Geometry: final body of the model. Coordinates: model frame, mm. Give positions to 0.01 mm unless a question says otherwise; leave off trailing zeros. Loops run counter-clockwise (first coordinate to the right, second up) from the corner with the lowest first, then second, coordinate; pieces in that order, holes last. Notation, with made-up numbers: (-26.75, 34.25) - (11.25, 34.25) arc R23 cw to (11.25, 49.25) - close; hole circle Ø5 at (65, 67). An arc over 180 degrees is marked (long way). Use one line per item in the form item = value.
Autodesk Inventor part; units mm, degrees
ref_plane "YZ Plane" through (0, 0, 0) normal (1, 0, 0) x (0, 1, 0)
ref_plane "XZ Plane" through (0, 0, 0) normal (0, 1, 0) x (-1, 0, 0)
ref_plane "XY Plane" through (0, 0, 0) normal (0, 0, 1) x (1, 0, 0)
sketch "Skizze1" plane through (0, 0, 0) normal (0, 0, 1) x (1, 0, 0)
  line L0 (0, 0) -> (90.4, 0)
  line L1 (90.4, 0) -> (90.4, 80)
  line L2 (90.4, 80) -> (0, 80)
  line L3 (0, 80) -> (0, 0)
  line L4 (2.6, 69.1) -> (87.8, 69.1) construction
  line L5 (87.8, 69.1) -> (87.8, 10.9) construction
  line L6 (87.8, 10.9) -> (2.6, 10.9) construction
  line L7 (2.6, 10.9) -> (2.6, 69.1) construction
  circle A0 centre (2.6, 69.1) radius 1.6
  circle A1 centre (2.6, 10.9) radius 1.6
  circle A2 centre (87.8, 69.1) radius 1.6
  circle A3 centre (87.8, 10.9) radius 1.6
  line L8 (25.2, 40) -> (65.2, 40) construction
  line L9 (65.2, 69.1) -> (65.2, 10.9) construction
  line L10 (65.2, 10.9) -> (47.65, 10.9) construction
  line L11 (65.2, 69.1) -> (82.75, 69.1) construction
  line L12 (25.2, 69.1) -> (25.2, 10.9) construction
  line L13 (25.2, 69.1) -> (42.75, 69.1) construction
  line L14 (25.2, 10.9) -> (7.65, 10.9) construction
  circle A4 centre (7.65, 10.9) radius 1.225
  circle A5 centre (42.75, 69.1) radius 1.225
  circle A6 centre (82.75, 69.1) radius 1.225
  circle A7 centre (47.65, 10.9) radius 1.225
  circle A8 centre (47.65, 77.32) radius 1.195
  circle A9 centre (42.75, 2.68) radius 1.195
  circle A10 centre (65.2, 10.9) radius 1.6
  circle A11 centre (65.2, 69.1) radius 1.6
  circle A12 centre (25.2, 69.1) radius 1.6
  circle A13 centre (25.2, 10.9) radius 1.6
  line L15 (1.9, 19.45) -> (3.9, 19.45) construction
  line L16 (3.9, 19.45) -> (3.9, 17.45) construction
  line L17 (3.9, 17.45) -> (1.9, 17.45) construction
  line L18 (1.9, 17.45) -> (1.9, 19.45) construction
  line L19 (1.9, 25.15) -> (3.9, 25.15) construction
  line L20 (3.9, 25.15) -> (3.9, 23.15) construction
  line L21 (3.9, 23.15) -> (1.9, 23.15) construction
  line L22 (1.9, 23.15) -> (1.9, 25.15) construction
  line L23 (1.8, 30.1) -> (4.2, 30.1) construction
  line L24 (4.2, 30.1) -> (4.2, 27.9) construction
  line L25 (4.2, 27.9) -> (1.8, 27.9) construction
  line L26 (1.8, 27.9) -> (1.8, 30.1) construction
  line L27 (2.9, 19.45) -> (2.9, 23.15) construction
  circle A14 centre (1.9, 23.15) radius 0.5588
  circle A15 centre (3.9, 23.15) radius 0.5588
  circle A16 centre (3.9, 25.15) radius 0.5588
  circle A17 centre (1.9, 25.15) radius 0.5588
  circle A18 centre (1.9, 19.45) radius 0.5588
  circle A19 centre (3.9, 19.45) radius 0.5588
  circle A20 centre (3.9, 17.45) radius 0.5588
  circle A21 centre (1.9, 17.45) radius 0.5588
  line L28 (1.8, 27.9) -> (4.2, 30.1) construction
  circle A22 centre (4.2, 27.9) radius 0.4064
  circle A23 centre (1.8, 27.9) radius 0.4064
  circle A24 centre (4.2, 30.1) radius 0.4064
  circle A25 centre (1.8, 30.1) radius 0.4064
  line L29 (86.3, 19.45) -> (88.3, 19.45) construction
  line L30 (88.3, 19.45) -> (88.3, 17.45) construction
  line L31 (88.3, 17.45) -> (86.3, 17.45) construction
  line L32 (86.3, 17.45) -> (86.3, 19.45) construction
  line L33 (86.3, 25.15) -> (88.3, 25.15) construction
  line L34 (88.3, 25.15) -> (88.3, 23.15) construction
  line L35 (88.3, 23.15) -> (86.3, 23.15) construction
  line L36 (86.3, 23.15) -> (86.3, 25.15) construction
  line L37 (87.3, 19.45) -> (87.3, 23.15) construction
  circle A26 centre (86.3, 23.15) radius 0.5588
  circle A27 centre (88.3, 23.15) radius 0.5588
  circle A28 centre (88.3, 25.15) radius 0.5588
  circle A29 centre (86.3, 25.15) radius 0.5588
  circle A30 centre (86.3, 19.45) radius 0.5588
  circle A31 centre (88.3, 19.45) radius 0.5588
  circle A32 centre (88.3, 17.45) radius 0.5588
  circle A33 centre (86.3, 17.45) radius 0.5588
  line L38 (55.65, 77.61) -> (74.75, 77.61) construction
  line L39 (74.75, 77.61) -> (74.75, 2.39) construction
  line L40 (74.75, 2.39) -> (55.65, 2.39) construction
  line L41 (55.65, 2.39) -> (55.65, 77.61) construction
  circle A34 centre (55.65, 2.39) radius 0.66
  circle A35 centre (74.75, 2.39) radius 0.66
  circle A36 centre (74.75, 77.61) radius 0.66
  circle A37 centre (55.65, 77.61) radius 0.66
  line L42 (15.65, 77.61) -> (34.75, 77.61) construction
  line L43 (34.75, 77.61) -> (34.75, 2.39) construction
  line L44 (34.75, 2.39) -> (15.65, 2.39) construction
  line L45 (15.65, 2.39) -> (15.65, 77.61) construction
  circle A38 centre (15.65, 2.39) radius 0.66
  circle A39 centre (34.75, 2.39) radius 0.66
  circle A40 centre (34.75, 77.61) radius 0.66
  circle A41 centre (15.65, 77.61) radius 0.66
  line L46 (55.65, 2.39) -> (74.75, 77.61) construction
  line L47 (15.65, 2.39) -> (34.75, 77.61) construction
  line L48 (23.2, 29.27) -> (23.2, 26.73) construction
  circle A42 centre (23.2, 26.73) radius 0.45
  circle A43 centre (23.2, 29.27) radius 0.45
  line L49 (27.2, 29.27) -> (27.2, 26.73) construction
  circle A44 centre (27.2, 26.73) radius 0.45
  circle A45 centre (27.2, 29.27) radius 0.45
  line L50 (23.2, 28) -> (27.2, 28) construction
  line L51 (63.2, 29.27) -> (63.2, 26.73) construction
  circle A46 centre (63.2, 26.73) radius 0.45
  circle A47 centre (63.2, 29.27) radius 0.45
  circle A48 centre (67.2, 29.27) radius 0.45
  line L52 (67.2, 29.27) -> (67.2, 26.73) construction
  circle A49 centre (67.2, 26.73) radius 0.45
  line L53 (63.2, 28) -> (67.2, 28) construction
  point P0 (2.9, 21.3)
  point P1 (3, 29)
  point P2 (87.3, 21.3)
  dimension "d0" = 90.4
  dimension "d1" = 80
  dimension "d2" = 2.6
  dimension "d3" = 10.9
  dimension "d4" = 69.1
  dimension "d5" = 87.8
  dimension "d6" = 3.2
  dimension "d7" = 40
  dimension "d8" = 25.2
  dimension "d9" = 65.2
  dimension "d10" = 2.45
  dimension "d11" = 2.39
  dimension "d12" = 17.55
  dimension "d13" = 17.55
  dimension "d14" = 37.32
  dimension "d15" = 37.32
  dimension "d16" = 3.2
  dimension "d17" = 29.1
  dimension "d18" = 17.55
  dimension "d21" = 1.85
  dimension "d22" = 2
  dimension "d23" = 1.1176
  dimension "d24" = 2.4
  dimension "d25" = 2.2
  dimension "d26" = 0.8128
  dimension "d27" = 1.85
  dimension "d28" = 2
  dimension "d29" = 1.1176
  dimension "d30" = 2.9
  dimension "d31" = 3
  dimension "d32" = 21.3
  dimension "d33" = 29
  dimension "d34" = 87.3
  dimension "d35" = 21.3
  dimension "d36" = 1.32
  dimension "d37" = 19.1
  dimension "d38" = 75.22
  dimension "d39" = 1.32
  dimension "d40" = 19.1
  dimension "d41" = 75.22
  dimension "d42" = 0.9
  dimension "d43" = 2.54
  dimension "d44" = 0.9
  dimension "d45" = 2.54
  dimension "d46" = 4
  dimension "d47" = 0.9
  dimension "d48" = 2.54
  dimension "d49" = 0.9
  dimension "d50" = 2.54
  dimension "d51" = 4
  dimension "d52" = 28
  dimension "d53" = 23.2
  dimension "d54" = 63.2
extrude "Extrusion1" add sketch "Skizze1" along normal mid plane 1.6
sketch "Skizze2" plane through (0, 0, 0.8) normal (0, 0, 1) x (1, 0, 0)
  line L0 (0, 79.9165) -> (90.4, 79.9165) construction
  line L1 (90.4, 79.9165) -> (90.4, 0.0835) construction
  line L2 (90.4, 0.0835) -> (0, 0.0835) construction
  line L3 (0, 0.0835) -> (0, 79.9165) construction
  point P0 (90.4, 40)
  point P1 (0, 40)
decal "Aufkleber1"
equation "\"d13\" = d12"
equation "\"d15\" = d14"
properties part number "PSU-PCB"
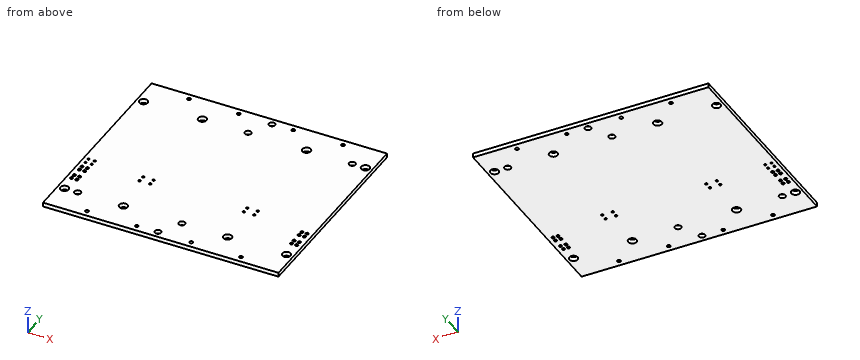
(1) Cut plane C-C (y = 69.1). Return the cut outline in (x, z) (3 decimals).
Solution:
outline = (0, -0.8) - (1, -0.8) - (1, 0.8) - (0, 0.8) - close; (4.2, -0.8) - (23.6, -0.8) - (23.6, 0.8) - (4.2, 0.8) - close; (26.8, -0.8) - (41.525, -0.8) - (41.525, 0.8) - (26.8, 0.8) - close; (43.975, -0.8) - (63.6, -0.8) - (63.6, 0.8) - (43.975, 0.8) - close; (66.8, -0.8) - (81.525, -0.8) - (81.525, 0.8) - (66.8, 0.8) - close; (83.975, -0.8) - (86.2, -0.8) - (86.2, 0.8) - (83.975, 0.8) - close; (89.4, -0.8) - (90.4, -0.8) - (90.4, 0.8) - (89.4, 0.8) - close
(2) Cut plane A-A (x = 82.75). Return the cut outline in (y, z) (3 decimals), plus the area to 3 significant figures.
Solution:
outline = (0, -0.8) - (67.875, -0.8) - (67.875, 0.8) - (0, 0.8) - close; (70.325, -0.8) - (80, -0.8) - (80, 0.8) - (70.325, 0.8) - close
area = 124 mm2
(3) Cut plane B-B (x = 42.75). Return the cut outline in (y, z) (3 decimals).
Solution:
outline = (0, -0.8) - (1.485, -0.8) - (1.485, 0.8) - (0, 0.8) - close; (3.875, -0.8) - (67.875, -0.8) - (67.875, 0.8) - (3.875, 0.8) - close; (70.325, -0.8) - (80, -0.8) - (80, 0.8) - (70.325, 0.8) - close
(4) Material intervals for L1, parallel to Y at x = 15.5, z = 0.7; L2, parallel to X at y = 19, z = 0.65; L3, parallel to X at y = 27, z = 0.7, sorted ascending. Write a range as from..to.
Solution:
L1 = 0..1.75, 3.03..76.97, 78.25..80
L2 = 0..1.57, 2.23..3.57, 4.23..85.97, 86.63..87.97, 88.63..90.4
L3 = 0..22.84, 23.56..26.84, 27.56..62.84, 63.56..66.84, 67.56..90.4
(5) Cut plane D-D (z = -0.25). Give the number of separate pieces and of enclosed holes in the cut face, plus the area to 3 significant figures.
Solution:
separate_pieces = 1
enclosed_holes = 50
area = 7,110 mm2
